Geometry check sheet. Reference: the model listing, model coordinates, mm. Give positions to 0.01 mm unless a question says otherwise; leave off trailing zeros. Write each loop counter-clockwise with the first axis right and the second up, starting at its lowest first coordinate (ties: lowest second). Pieces come first, ordered by that corner, then holes. Notation, with made-up numbers: (-22, 48) -> (29, 48) arc R18 cw to (29, 68) -> close; hole circle Ø11 at (-3.5, -18.75). An arc over 180 degrees is marked (long way). One line per item, written item: value.
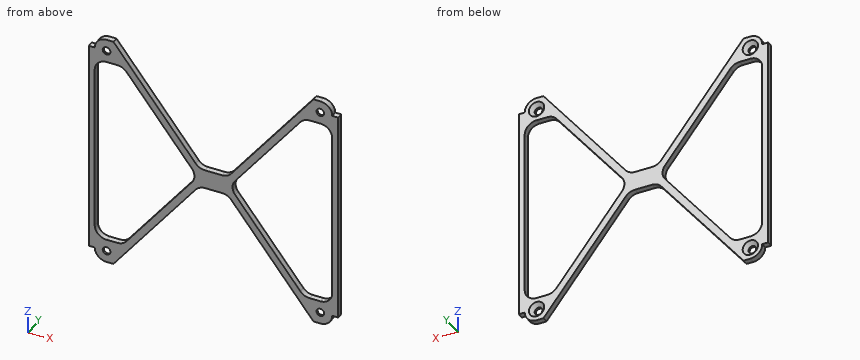
from build123d import *

# Parameters (mm, degrees)
SKETCH1_R           = 1.625
BOSS_EXTRUDE1_DEPTH = 2.5
FILLET1_R           = 5
FILLET2_R           = 5
CHAMFER1_SIZE       = 1.6


with BuildPart() as part:
    # Sketch1 → Boss-Extrude1 (new body)
    with BuildSketch(Plane(origin=(0, 0, 0), x_dir=(1, 0, 0), z_dir=(0, 1, 0))):
        with BuildLine():
            Line((-52.5, 45), (-52.5, -45))
            Line((-52.5, -45), (-50, -45))
            ThreePointArc((-50, -45), (-48.535533906, -48.535533906), (-45, -50))
            Line((-45, -50), (-42.127158908, -50))
            Line((-42.127158908, -50), (-6, -4))
            Line((-6, -4), (6, -4))
            Line((6, -4), (42.127158908, -50))
            Line((42.127158908, -50), (45, -50))
            ThreePointArc((45, -50), (48.535533906, -48.535533906), (50, -45))
            Line((50, -45), (52.5, -45))
            Line((52.5, -45), (52.5, 45))
            Line((52.5, 45), (50, 45))
            ThreePointArc((50, 45), (48.535533906, 48.535533906), (45, 50))
            Line((45, 50), (42.127158908, 50))
            Line((42.127158908, 50), (6, 4))
            Line((6, 4), (-6, 4))
            Line((-6, 4), (-42.127158908, 50))
            Line((-42.127158908, 50), (-45, 50))
            ThreePointArc((-45, 50), (-48.535533906, 48.535533906), (-50, 45))
            Line((-50, 45), (-52.5, 45))
        make_face()
        with Locations(Location((-45, 45, 0), (0, 0, 270))):
            Circle(SKETCH1_R, mode=Mode.SUBTRACT)
        with Locations(Location((45, 45, 0), (0, 0, 270))):
            Circle(SKETCH1_R, mode=Mode.SUBTRACT)
        with Locations(Location((-45, -45, 0), (0, 0, 270))):
            Circle(SKETCH1_R, mode=Mode.SUBTRACT)
        with Locations(Location((45, -45, 0), (0, 0, 270))):
            Circle(SKETCH1_R, mode=Mode.SUBTRACT)
        Polygon((-50, 40), (-50, -40), (-38.088044946, -40), (-6.673124156, 0), (-38.088044946, 40), align=None, mode=Mode.SUBTRACT)
        Polygon((50, -40), (38.088044946, -40), (6.673124156, 0), (38.088044946, 40), (50, 40), align=None, mode=Mode.SUBTRACT)
    extrude(amount=BOSS_EXTRUDE1_DEPTH)

    # Fillet1
    fillet1_edges = [part.edges().sort_by_distance(p)[0] for p in [
        (-6, 1.25, -4),
        (6, 1.25, -4),
        (6, 1.25, 4),
        (-6, 1.25, 4),
        (-6.673124156, 1.25, 0),
        (6.673124156, 1.25, 0),
    ]]
    fillet(fillet1_edges, radius=FILLET1_R)

    # Fillet2
    fillet2_edges = [part.edges().sort_by_distance(p)[0] for p in [
        (-38.088044946, 1.25, -40),
        (-50, 1.25, -40),
        (-50, 1.25, 40),
        (-38.088044946, 1.25, 40),
        (50, 1.25, 40),
        (50, 1.25, -40),
        (38.088044946, 1.25, -40),
        (38.088044946, 1.25, 40),
    ]]
    fillet(fillet2_edges, radius=FILLET2_R)

    # Chamfer1
    chamfer1_edges = [part.edges().sort_by_distance(p)[0] for p in [
        (-45, 2.5, -46.625),
        (45, 2.5, -46.625),
        (-45, 2.5, 43.375),
        (45, 2.5, 43.375),
    ]]
    chamfer(chamfer1_edges, length=CHAMFER1_SIZE)


solid = part.part
1) Sectioned sample at A-A on x = 20.5. Record the cut outline in (y, z), plus the area to 3 significant figures.
Verdict:
outline: (0, -22.46) -> (2.5, -22.46) -> (2.5, -17.61) -> (0, -17.61) -> close; (0, 17.61) -> (2.5, 17.61) -> (2.5, 22.46) -> (0, 22.46) -> close
area: 24.3 mm^2
2) Scan lines: probe 1 along X at (y, z) = (0.75, -4.5); probe 2 along X at (y, z) = (1.65, -13); probe 3 along Z at (x, y) = (-21, 1.3). Record each from-to range of solid material in increasing order.
Verdict:
probe 1: -52.5 to -50, -10.21 to -5.75, 5.75 to 10.21, 50 to 52.5
probe 2: -52.5 to -50, -16.88 to -13.07, 13.07 to 16.88, 50 to 52.5
probe 3: -23.1 to -18.24, 18.24 to 23.1
3) Depth check by flat-ended pin: pin 1 Ø1.5 at (x, y) = (-37.5, 1) entering from -Z; pin 2 Ø1.2 at (x, y) = (-52, 0.5) entering from +Z; pin 3 Ø1.2 at (x, y) = (-1, 1) entering from -Z; pin 4 Ø1.9 at (x, z) = (45, 45) entering from +Y. Enter the tip coordinate at first touch or a pass-through.
Verdict:
pin 1: z = -45.06
pin 2: z = 45
pin 3: z = -4
pin 4: through
4) Sectioned sample at C-C on x = -5.5. Record the cut outline in (y, z).
Verdict:
outline: (0, -4.39) -> (2.5, -4.39) -> (2.5, 4.39) -> (0, 4.39) -> close
5) Sectioned sample at B-B on x = 38.5. Record the cut outline in (y, z).
Verdict:
outline: (0, -45.38) -> (2.5, -45.38) -> (2.5, -39.57) -> (0, -39.57) -> close; (0, 39.57) -> (2.5, 39.57) -> (2.5, 45.38) -> (0, 45.38) -> close
